Read the model definition and answer for the solid it produces. Units are mm, in the model's axes. A direction names the side the tool comes from. Coordinates: 2 decimals unless noted, no trailing zeros. Loops run counter-clockwise (first coordinate to the right, second up) from the corner with the lowest first, then second, coordinate; pieces in that order, holes last. Notation, with made-up numbers: (57.25, 48) - (83.25, 48) arc R29 cw to (83.25, 82) - close; hole circle Ø10 at (-20.5, -38). An arc over 180 degrees is marked (long way). Use one line per item in the form item = value.
from build123d import *

# Parameters (mm, degrees)
SKETCH_1_R          = 25
EXTRUDE_1_DEPTH     = 5
SKETCH_2_R          = 2.5
EXTRUDE_2_DEPTH     = 7
SKETCH_3_W          = 2
SKETCH_3_H          = 2
CUT_EXTRUDE_1_DEPTH = 37.041642582


with BuildPart() as part:
    # 草图1 → 凸台-拉伸1 (new body)
    with BuildSketch(Plane.XY):
        Circle(SKETCH_1_R)
    extrude(amount=EXTRUDE_1_DEPTH)

    # 草图2 → 凸台-拉伸2 (add)
    with BuildSketch(Plane.XY.offset(5)):
        with Locations((-20, 0)):
            Circle(SKETCH_2_R)
    extrude(amount=EXTRUDE_2_DEPTH)

    # 草图3 → 切除-拉伸1 (cut, through all)
    with BuildSketch(Plane.XY.offset(5)):
        with Locations((0, 2)):
            Rectangle(SKETCH_3_W, SKETCH_3_H)
        with Locations((-2, 0)):
            Rectangle(SKETCH_3_W, SKETCH_3_H)
        with Locations((2, 0)):
            Rectangle(SKETCH_3_W, SKETCH_3_H)
        with Locations((0, -2)):
            Rectangle(SKETCH_3_W, SKETCH_3_H)
        Rectangle(SKETCH_3_W, SKETCH_3_H)
    extrude(amount=-CUT_EXTRUDE_1_DEPTH, mode=Mode.SUBTRACT)


solid = part.part
Item 1: Which of the six approach directions +Z, -Z, +X, -X, +Y, -Y give full straight-line access (tool end or side, diameter ignored) to faces 4 (the flat face through (-20, 0, 12)), 5 (the cylindrical face through (-22.5, 0.1, 8.5)), 6 (the flat face through (-1, -2, 3))?
Results below:
face_4 = +Z, +X, -X, +Y, -Y
face_5 = +Z
face_6 = +Z, -Z
Item 2: Find the intervals of material crossed by L1, parallel to Z at x = 13.5, y = -8.5; L2, parallel to Y at x = -0.5, z = 1 (3 decimals); L3, parallel to Y at x = 2, z = 0.5, in increasing order.
Results below:
L1 = 0 to 5
L2 = -24.995 to -3, 3 to 24.995
L3 = -24.92 to -1, 1 to 24.92
Item 3: The part is cut by section C-C on z = 2.25. Give the vertices of the cut face in (x, y), plus the area to 3 significant figures.
Results below:
outline = circle Ø50 at (0, 0); hole (-3, -1) - (-1, -1) - (-1, -3) - (1, -3) - (1, -1) - (3, -1) - (3, 1) - (1, 1) - (1, 3) - (-1, 3) - (-1, 1) - (-3, 1) - close
area = 1,940 mm²
Item 4: The part is cut by section D-D on x = -20. Give the vertices of the cut face in (y, z).
Results below:
outline = (-15, 0) - (15, 0) - (15, 5) - (2.5, 5) - (2.5, 12) - (-2.5, 12) - (-2.5, 5) - (-15, 5) - close
Item 5: The part is cut by section B-B on x = 0. Give the vertices of the cut face in (y, z), plus the area to 3 significant figures.
Results below:
outline = (-25, 0) - (-3, 0) - (-3, 5) - (-25, 5) - close; (3, 0) - (25, 0) - (25, 5) - (3, 5) - close
area = 220 mm²
Item 6: The part is cut by section A-A on y = 0. Give the vertices of the cut face in (x, z).
Results below:
outline = (-25, 0) - (-3, 0) - (-3, 5) - (-17.5, 5) - (-17.5, 12) - (-22.5, 12) - (-22.5, 5) - (-25, 5) - close; (3, 0) - (25, 0) - (25, 5) - (3, 5) - close
Item 7: For a pull along X with two mould halves and no side action, classify faces 1 (the flat face through (0, -5, 0)), 2 (the flat face through (3, 0, 3)), 3 (the cylindrical face through (23.846, 7.509, 2.465)) as +X half, -X half, draft (parallel to the pull), parting line (faces both ways), or undercut.
Results below:
face_1 = draft
face_2 = undercut
face_3 = parting line
Item 8: Each of these flat-tipped pins is pushed along its axis until it touches: P1, Ø0.6, axis at x = 2, z = 3, coming from the -Y side; P2, Ø0.6, axis at y = -2, z = 2, coming from the +X side; P3, Ø0.6, axis at y = 1.5, z = 2.5, coming from the +X side. Where does it stop, or does it pass through?
Results below:
P1 = -24.94
P2 = 24.94
P3 = 24.97
